Autodesk Inventor part; units mm, degrees
ref_plane "YZ Plane" through (0, 0, 0) normal (1, 0, 0) x (0, 1, 0)
ref_plane "XZ Plane" through (0, 0, 0) normal (0, 1, 0) x (-1, 0, 0)
ref_plane "XY Plane" through (0, 0, 0) normal (0, 0, 1) x (1, 0, 0)
sketch "Эскиз1" plane through (0, 0, 0) normal (0, 1, 0) x (-1, 0, 0)
  line L0 (0, 0) -> (10, 0)
  line L1 (10, 0) -> (10, -30)
  line L2 (10, -30) -> (0, -30)
  line L3 (0, -30) -> (0, 0)
  dimension "d0" = 10
  dimension "d1" = 30
extrude "Выдавливание1" add sketch "Эскиз1" along normal blind 20
sketch "Эскиз2" plane through (0, 20, 0) normal (0, 1, 0) x (1, 0, 0)
  line L0 (-7.0207, 11.5) -> (-9.0415, 15)
  line L1 (-9.0415, 15) -> (-7.0207, 18.5)
  line L2 (-7.0207, 18.5) -> (-2.9793, 18.5)
  line L3 (-2.9793, 18.5) -> (-0.9585, 15)
  line L4 (-0.9585, 15) -> (-2.9793, 11.5)
  line L5 (-2.9793, 11.5) -> (-7.0207, 11.5)
  line L6 (-10, 30) -> (-10, 0)
  line L7 (0, 30) -> (-10, 30)
  point P0 (0, 0)
  point P1 (-5, 15)
  point P2 (-10, 15)
  point P3 (-5, 30)
  dimension "d4" = 3.5
sketch "Эскиз3" plane through (0, 20, 0) normal (0, 1, 0) x (1, 0, 0)
  circle A0 centre (-5, 15) radius 2
  point P0 (0, 0)
  dimension "d5" = 4
extrude "Выдавливание2" cut sketch "Эскиз3" against normal blind 10
extrude "Выдавливание3" cut sketch "Эскиз2" against normal blind 3.2
properties part number "FlanecPodGayku"
Work out the finished part from the listing and answer in its coordinate system (mm). A direction names the side the tool comes from. Give positions to 0.01 mm unless a question says otherwise; leave off trailing zeros. Write each loop counter-clockwise with the first axis right and the second up, starting at its lowest first coordinate (ties: lowest second). Pieces come first, ordered by that corner, then holes. Notation, with made-up numbers: M 63,-2 L 91,-2 A22 cw 91,36 Z; hole C 66.5,9 d4. An arc over 180 degrees is marked long. Answer as CSV lines item,"result".
Q1. Given P1, Ø1, axis at x = -7, z = -16, coming from the +Y side; P2, Ø1.2, axis at x = -5.5, z = -14.5, coming from the +Y side, each flat-ended and moving along its own axis, determine where each tip first touches the part or whether it passes through.
A:
P1,"stops at y = 16.8"
P2,"stops at y = 10"
Q2. The mould has two halves that part along X. Classify faces 3 (the flat face through (-1.955, 18.422, -13.274)), 4 (the flat face through (-5, 20, -11)), 5 (the flat face through (-2, 18.4, -16.8)), 6 (the flat face through (0, 10, -15)): +X half, -X half, draft (parallel to the pull), parting line (faces both ways), or undercut.
A:
face 3,"undercut"
face 4,"draft"
face 5,"undercut"
face 6,"+X half"
Q3. A cutting plane is placed at A-A on y = 18.5. Write down the section's boundary in (x, z), plus the area to 3 significant figures.
A:
outline,"M -10,-30 L 0,-30 L 0,0 L -10,0 Z; hole M -9.04,-15 L -7.02,-18.5 L -2.98,-18.5 L -0.96,-15 L -2.98,-11.5 L -7.02,-11.5 Z"
area,"258 mm²"
Q4. A cutting plane is placed at D-D on y = 13.5. Write down the section's boundary in (x, z).
A:
outline,"M -10,-30 L 0,-30 L 0,0 L -10,0 Z; hole C -5,-15 d4"
Q5. Find the intervals of material crossed by probe 1 along Z at (x, y) = (-5, 15.25); probe 2 along X at (y, z) = (14, -15); probe 3 along Y at (x, z) = (-3, -15.5), in increasing order. Write a range as [from, to].
A:
probe 1,"z = [-30, -17], [-13, 0]"
probe 2,"x = [-10, -7], [-3, 0]"
probe 3,"y = [0, 16.8]"
Q6. A cutting plane is placed at B-B on x = -5. Write down the section's boundary in (y, z).
A:
outline,"M 0,-30 L 20,-30 L 20,-18.5 L 16.8,-18.5 L 16.8,-17 L 10,-17 L 10,-13 L 16.8,-13 L 16.8,-11.5 L 20,-11.5 L 20,0 L 0,0 Z"
Q7. A tool of negligible diameter and unlimited length cuts with its end or side. For faces 1 (the flat face through (-5, 18, -11.5)), 2 (the flat face through (-10, 10, -15)), from which of +Z, -Z, +X, -X, +Y, -Y can it reach the whole face along a straight path? Write none if from no direction.
A:
face 1,"+Y"
face 2,"+Z, -Z, -X, +Y, -Y"
Q8. A cutting plane is placed at C-C on z = -16. Write down the section's boundary in (x, y).
A:
outline,"M -10,0 L 0,0 L 0,20 L -1.54,20 L -1.54,16.8 L -3.27,16.8 L -3.27,10 L -6.73,10 L -6.73,16.8 L -8.46,16.8 L -8.46,20 L -10,20 Z"
